Part model, mm, in its own coordinate system. Face numbers are marked on the shaded views. A direction names the side the tool comes from. Round coordinates to 2 decimals unless told otherwise and drop trailing zeros. Write each loop counter-clockwise with the first axis right and the second up, starting at its lowest first coordinate (ties: lowest second). Pieces come first, ordered by that corner, then holes.
```python
from build123d import *

# Parameters (mm, degrees)
SKETCH_1_W          = 23
SKETCH_1_H          = 12
EXTRUDE_1_DEPTH     = 24
SKETCH_2_W          = 12
SKETCH_2_H          = 2.5
EXTRUDE_2_DEPTH     = 5
SKETCH_3_W          = 12
SKETCH_3_H          = 2.5
EXTRUDE_3_DEPTH     = 5
SKETCH_4_R          = 6
EXTRUDE_4_DEPTH     = 4
SKETCH_5_R          = 2.5
EXTRUDE_5_DEPTH     = 3
SKETCH_6_R          = 1.25
CUT_EXTRUDE_1_DEPTH = 3


with BuildPart() as part:
    # 草图1 → 凸台-拉伸1 (new body)
    with BuildSketch(Plane(origin=(0, 0, 0), x_dir=(1, 0, 0), z_dir=(0, 1, 0))):
        Rectangle(SKETCH_1_W, SKETCH_1_H)
    extrude(amount=EXTRUDE_1_DEPTH)

    # 草图2 → 凸台-拉伸2 (add)
    with BuildSketch(Plane(origin=(11.5, 0, 0), x_dir=(0, 0, -1), z_dir=(1, 0, 0))):
        with Locations((0, 18.25)):
            Rectangle(SKETCH_2_W, SKETCH_2_H)
    extrude(amount=EXTRUDE_2_DEPTH)

    # 草图3 → 凸台-拉伸3 (add)
    with BuildSketch(Plane.ZY.offset(11.5)):
        with Locations((0, 18.25)):
            Rectangle(SKETCH_3_W, SKETCH_3_H)
    extrude(amount=EXTRUDE_3_DEPTH)

    # 草图4 → 凸台-拉伸4 (add)
    with BuildSketch(Plane(origin=(0, 24, 0), x_dir=(1, 0, 0), z_dir=(0, 1, 0))):
        with Locations(Location((5.5, 0, 0), (0, 0, 270))):
            Circle(SKETCH_4_R)
    extrude(amount=EXTRUDE_4_DEPTH)

    # 草图5 → 凸台-拉伸5 (add)
    with BuildSketch(Plane(origin=(0, 28, 0), x_dir=(1, 0, 0), z_dir=(0, 1, 0))):
        with Locations(Location((5.5, 0, 0), (0, 0, 270))):
            Circle(SKETCH_5_R)
    extrude(amount=EXTRUDE_5_DEPTH)

    # 草图6 → 切除-拉伸1 (cut)
    with BuildSketch(Plane(origin=(0, 19.5, 0), x_dir=(1, 0, 0), z_dir=(0, 1, 0))):
        with Locations(Location((13.75, 0, 0), (0, 0, 270))):
            Circle(SKETCH_6_R)
        with Locations(Location((-13.75, 0, 0), (0, 0, 270))):
            Circle(SKETCH_6_R)
    extrude(amount=-CUT_EXTRUDE_1_DEPTH, mode=Mode.SUBTRACT)


solid = part.part
```
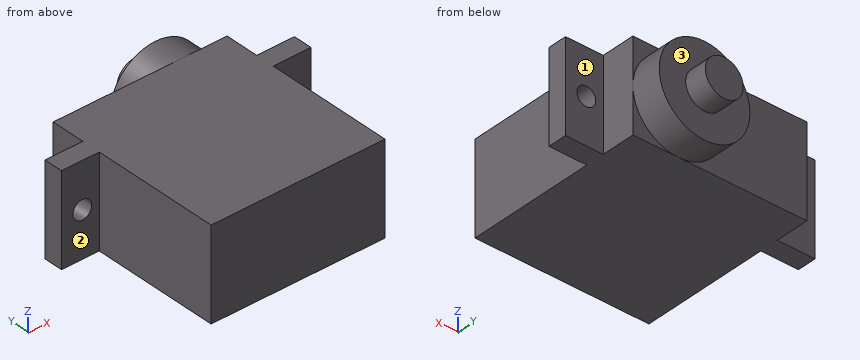
Q1. Drop flat-ended pins along their axis: pin 1 (5 mm diameter, centred on y = 22.5, z = -1, fed in from -X); pin 2 (3 mm diameter, centred on x = 9.5, z = 2, fed in from +Y); pin 3 (4 mm diameter, centred on x = 14, z = 0, fed in from +Y). Give the stop position or say it passes through.
Values follow:
pin 1: stops at x = -11.5
pin 2: stops at y = 28
pin 3: stops at y = 19.5
Q2. Which spindle directions (+Z, -Z, +X, -X, +Y, -Y) get a long thin tool onto all of the face, cutting with end or side? Do the marked faces 1, 2 and 3. Say none if no direction does.
Values follow:
face 1: +Z, -Z, +X, +Y
face 2: +Z, -Z, -X, -Y
face 3: +Y
Q3. Cut at B-B on z = 5.25. Write the cut outline in (x, y).
Values follow:
outline: (-16.5, 17) - (-11.5, 17) - (-11.5, 0) - (11.5, 0) - (11.5, 17) - (16.5, 17) - (16.5, 19.5) - (11.5, 19.5) - (11.5, 24) - (8.4, 24) - (8.4, 28) - (2.6, 28) - (2.6, 24) - (-11.5, 24) - (-11.5, 19.5) - (-16.5, 19.5) - close
Q4. Cut at A-A on x = -13.75. Write the cut outline in (y, z), plus the area to 4 significant figures.
Values follow:
outline: (17, -6) - (19.5, -6) - (19.5, -1.25) - (17, -1.25) - close; (17, 1.25) - (19.5, 1.25) - (19.5, 6) - (17, 6) - close
area: 23.75 mm2
Q5. Cut at C-C on x = 9.5. Write the cut outline in (y, z), plus the area to 3 significant figures.
Values follow:
outline: (0, -6) - (24, -6) - (24, -4.47) - (28, -4.47) - (28, 4.47) - (24, 4.47) - (24, 6) - (0, 6) - close
area: 324 mm2
Q6. Cut at D-D on y = 27. Write the cut outline in (x, z).
Values follow:
outline: circle Ø12 at (5.5, 0)
Q7. Wall check: L1, parallel to X at y = 16, z = -4.5; L2, parallel to Y at x = 13, z = 2.75; L3, parallel to Z at x = 13, y = 18. Give the ranges that are in metal, low to high.
Values follow:
L1: x = -11.5 to 11.5
L2: y = 17 to 19.5
L3: z = -6 to -1, 1 to 6
